from build123d import *

# Parameters (mm, degrees)
SCHNITT_LINEAR_AUSTRAGEN1_DEPTH      = 50.749371855
SCHNITT_LINEAR_AUSTRAGEN1_DEPTH_BACK = 50.749371855
SKIZZE3_W                            = 6
SKIZZE3_H                            = 0.5
M4_GEWINDEBOHRUNG2_D                 = 3.3
M4_GEWINDEBOHRUNG2_DEPTH             = 8.5
M4_GEWINDEBOHRUNG2_TIP               = 0.991420021
SKIZZE10_W                           = 5.838792557
SKIZZE10_H                           = 2
SCHNITT_LINEAR_AUSTRAGEN2_DEPTH      = 2
VERRUNDUNG1_R                        = 1


with BuildPart() as part:
    # Skizze1 → Rotation1 (revolve)
    with BuildSketch(Plane.XY, mode=Mode.PRIVATE) as rotation1_sk:
        Polygon((0, 3.2), (10, 3.2), (11.922753981, 0), (45, 0), (45, 4), (15, 4), (15, 7.5), (2, 7.5), (2, 15), (0, 15), (0, 7.5), align=None)
    revolve(rotation1_sk.sketch.rotate(Axis((0, 0, 0), (1, 0, 0)), 90), axis=Axis((0, 0, 0), (1, 0, 0)))

    # Skizze3 → Schnitt-Linear austragen1 (cut, two sides: drawn at the far end of the back side and taken through both)
    with BuildSketch(Plane(origin=(0, 0, 0), x_dir=(1, 0, 0), z_dir=(0, 1, 0)).offset(-SCHNITT_LINEAR_AUSTRAGEN1_DEPTH_BACK)):
        with Locations((32, 3.75)):
            Rectangle(SKIZZE3_W, SKIZZE3_H)
    extrude(amount=SCHNITT_LINEAR_AUSTRAGEN1_DEPTH + SCHNITT_LINEAR_AUSTRAGEN1_DEPTH_BACK, mode=Mode.SUBTRACT)

    # M4 Gewindebohrung2
    with Locations(Plane(origin=(0, 0, -7.5), x_dir=(1, 0, 0), z_dir=(0, 0, -1))):
        with Locations((5, 0)):
            Hole(M4_GEWINDEBOHRUNG2_D / 2, depth=M4_GEWINDEBOHRUNG2_DEPTH)
            with Locations((0, 0, -(M4_GEWINDEBOHRUNG2_DEPTH + M4_GEWINDEBOHRUNG2_TIP / 2))):  # 118° drill point
                Cone(0, M4_GEWINDEBOHRUNG2_D / 2, M4_GEWINDEBOHRUNG2_TIP, mode=Mode.SUBTRACT)

    # Skizze10 → Schnitt-Linear austragen2 (cut)
    with BuildSketch(Plane.ZY):
        with Locations((12.919396279, 0)):
            Rectangle(SKIZZE10_W, SKIZZE10_H)
    extrude(amount=-SCHNITT_LINEAR_AUSTRAGEN2_DEPTH, mode=Mode.SUBTRACT)

    # Verrundung1
    verrundung1_edges = [part.edges().sort_by_distance(p)[0] for p in [
        (1, -1, 10),
        (1, 1, 10),
    ]]
    fillet(verrundung1_edges, radius=VERRUNDUNG1_R - 0.0001)  # a hair under: the kernel refuses the full size


solid = part.part
The model under review builds one solid part; all positions refer to its coordinate system, in mm. A direction names the side the tool comes from. Round coordinates to 2 decimals unless told otherwise and drop trailing zeros. Order: outer loops, then holes, each group sorted by start corner. A loop starts at its lowest first (then second) coordinate and runs counter-clockwise, first axis right, second up. Notation, with made-up numbers: (-14, 22.5) -> (-1, 22.5) arc R27 ccw to (-1, 49.5) -> close; hole circle Ø3 at (26.5, -27). An arc over 180 degrees is marked (long way). Return JSON: item names as keys, results as strings.
1. For L1, parallel to Y at x = 7, z = 0; L2, parallel to Y at x = 21, z = -3.5; L3, parallel to Y at x = 3, z = -1.75, list the stretches that pass through material, from the lowest coordinate up. Write a range as [from, to].
Answer block:
{"L1": "y = [-7.5, -3.2], [3.2, 7.5]", "L2": "y = [-1.94, 1.94]", "L3": "y = [-7.29, -2.68], [2.68, 7.29]"}
2. Take a section at C-C (z = -12). Write out the cut boundary in (x, y), then the cut area to 3 significant figures.
Answer block:
{"outline": "(0, -9) -> (2, -9) -> (2, 9) -> (0, 9) -> close", "area": "36.0 mm²"}
3. The part is to be moulded in two halves that separate along X. For faces 1 (the face through (0, -4, 0)), 2 (the face through (1.014, 0.699, 10.285)), 3 (the face through (32, 0, -3.5)), say which applies: +X half, -X half, draft (parallel to the pull), parting line (faces both ways), or undercut.
Answer block:
{"face 1": "-X half", "face 2": "draft", "face 3": "undercut"}
4. For faces 4 (the face through (1, -1, 13)), 5 (the face through (5.07, -0.961, 3.052)), 6 (the face through (15, 3, -3)), list the 3-axis set-ups (+Z, -Z, +X, -X, +Y, -Y) from which the entire face can be reached by the end or side of a thin tool; tool diameter is ignored.
Answer block:
{"face 4": "+Z, +X, -X", "face 5": "-X", "face 6": "+X"}
5. Take a section at A-A (z = -6). Write out the cut boundary in (x, y), then the cut area to 3 significant figures.
Answer block:
{"outline": "(0, -13.75) -> (2, -13.75) -> (2, -4.5) -> (15, -4.5) -> (15, 4.5) -> (2, 4.5) -> (2, 13.75) -> (0, 13.75) -> close; hole circle Ø3.3 at (5, 0)", "area": "163 mm²"}
6. Insertion check: P1, Ø8, axis at x = 39, y = 6, coming from the +Z side; P2, Ø1.2, axis at x = 33, y = 0, coming from the -Z side; P3, Ø3, axis at x = 27.5, y = -1.5, coming from the -Z side. Each pin has a flat end and moves straight along its axis. Give the tip position at first contact, or say it passes through.
Answer block:
{"P1": "stops at z = 3.46", "P2": "stops at z = -3.5", "P3": "stops at z = -4"}
7. Take a section at B-B (y = 6). Write out the cut boundary in (x, z).
Answer block:
{"outline": "(0, -13.75) -> (2, -13.75) -> (2, -4.5) -> (15, -4.5) -> (15, 4.5) -> (2, 4.5) -> (2, 13.75) -> (0, 13.75) -> close"}
8. Take a section at D-D (x = 31.5). Write out the cut boundary in (y, z), then the cut area to 3 significant figures.
Answer block:
{"outline": "(-1.94, -3.5) -> (1.94, -3.5) arc R4 ccw (long way) to start", "area": "49.0 mm²"}
